```python
from build123d import *

# Parameters (mm, degrees)
SKETCH1_R           = 171.45
SKETCH1_R_2         = 109.5375
BOSS_EXTRUDE1_DEPTH = 1.5875
SKETCH2_R           = 11.176
CUT_EXTRUDE1_DEPTH  = 243.472112121
CIRPATTERN1_COUNT   = 8


with BuildPart() as part:
    # Sketch1 → Boss-Extrude1 (new, symmetric)
    with BuildSketch(Plane.XY):
        Circle(SKETCH1_R)
        Circle(SKETCH1_R_2, mode=Mode.SUBTRACT)
    extrude(amount=BOSS_EXTRUDE1_DEPTH, both=True)

    # Sketch2 → Cut-Extrude1 (cut, symmetric)
    with BuildSketch(Plane.XY):
        with Locations((0, 149.225)):
            Circle(SKETCH2_R)
    cut_extrude1 = extrude(amount=CUT_EXTRUDE1_DEPTH, both=True, mode=Mode.SUBTRACT)

    # CirPattern1: Cut-Extrude1 ×8 about axis
    cirpattern1_axis = Axis((0, 0, 0), (0, 0, 1))
    for i in range(1, CIRPATTERN1_COUNT):
        add(cut_extrude1.rotate(cirpattern1_axis, i * 360 / CIRPATTERN1_COUNT), mode=Mode.SUBTRACT)


solid = part.part
```
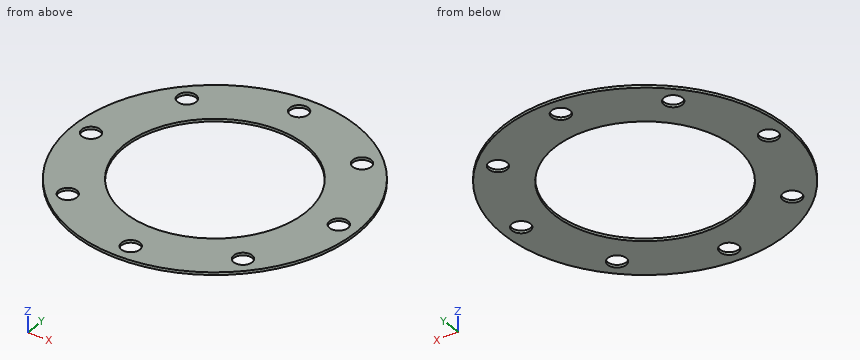
Check sheet for the modelled part. Datum: model origin and axes. Units: mm. Coordinates: 2 decimals unless noted, no trailing zeros. Loops run counter-clockwise (first coordinate to the right, second up) from the corner with the lowest first, then second, coordinate; pieces in that order, holes last.
1) Sectioned sample at D-D (z = -0.15). Count the separate pieces of the cut face and the enclosed holes in it, and give its area (3 significant figures).
2) Gauge pin test, flat ends, axial feed: pin 1 (13.5 mm diameter, centred on x = 149.225, y = 0, fed in from -Z); pin 2 (1 mm diameter, centred on y = 92.5, z = 0.5, fed in from +X). Record the tip position at first contact, or that the pin passes through.
3) Material ranges on probe 1 along Y at (x, z) = (0, -0.7); probe 2 along Y at (x, z) = (113, -0.9); probe 3 along X at (y, z) = (-10, 0.9), recorded low to high.
4) Sectioned sample at A-A (y = 0). Record the boundary of the cut face in (x, z), and give its area (3 significant figures).
5) Sectioned sample at C-C (y = 86.5). Record the boundary of the cut face in (x, z).
Check sheet entries:
1. separate pieces: 1
1. enclosed holes: 9
1. area: 51,500 mm2
2. pin 1: passes through
2. pin 2: stops at x = 144.68
3. probe 1: y = -171.45 to -160.4, -138.05 to -109.54, 109.54 to 138.05, 160.4 to 171.45
3. probe 2: y = -128.94 to -113.82, -97.22 to 97.22, 113.82 to 128.94
3. probe 3: x = -171.16 to -154.22, -144.23 to -109.08, 109.08 to 144.23, 154.22 to 171.16
4. outline: (-171.45, -1.59) - (-160.4, -1.59) - (-160.4, 1.59) - (-171.45, 1.59) - close; (-138.05, -1.59) - (-109.54, -1.59) - (-109.54, 1.59) - (-138.05, 1.59) - close; (109.54, -1.59) - (138.05, -1.59) - (138.05, 1.59) - (109.54, 1.59) - close; (160.4, -1.59) - (171.45, -1.59) - (171.45, 1.59) - (160.4, 1.59) - close
4. area: 251 mm2
5. outline: (-148.03, -1.59) - (-67.2, -1.59) - (-67.2, 1.59) - (-148.03, 1.59) - close; (67.2, -1.59) - (148.03, -1.59) - (148.03, 1.59) - (67.2, 1.59) - close
